The figure shows three views and two pictorial views of one solid part (mm, origin at its lowest corner). Answer the questions. A direction names the side the tool comes from. Coordinates: 2 decimals unless noted, no trailing zeros. Loops run counter-clockwise (first coordinate to the right, second up) from the corner with the lowest first, then second, coordinate; pieces in that order, holes last. Notation, with made-up numbers: M 16.5,74 L 31.5,74 A32 ccw 31.5,102 Z; hole C 49,-26.5 d10. An arc over 180 degrees is marked long. Answer as a JSON object with one key per item and string values. Group by question number.
1. A cutting plane is placed at B-B on y = 2. Give the vertices of the cut face in (x, z), and give its area (3 significant figures).
2. For the marked faces 1 and 2, determine the directions among +Z, -Z, +X, -X, +Y, -Y from which every point of the face is accessible in a straight line to the end or side of a thin tool.
3. A cutting plane is placed at A-A on y = 8.25. Give the vertices of the cut face in (x, z).
4. Straight lines are drawn through the part: L1, parallel to Y at x = 2.85, z = 1.65; L2, parallel to X at y = 5, z = 1.55; L3, parallel to X at y = 3, z = 1. For each, find the intervals that lie inside material, in ascending order.
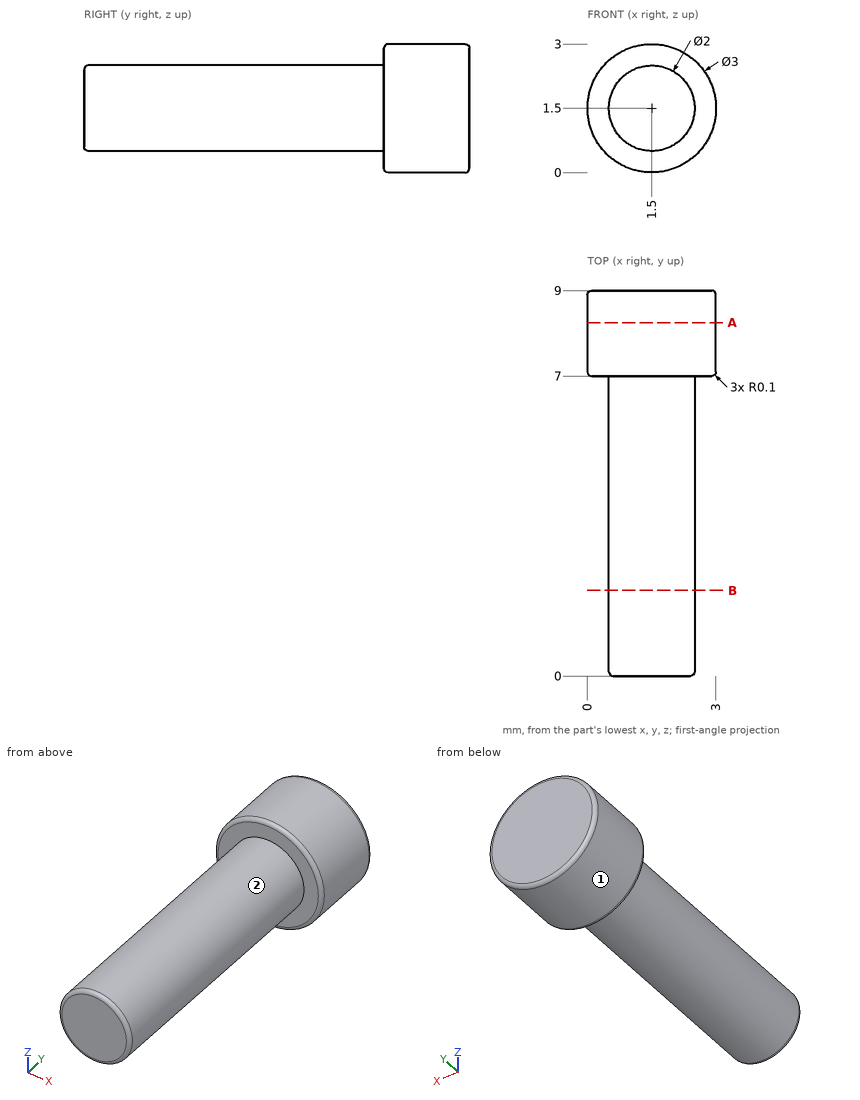
From the geometry:
{
 "1": {"outline": "C 1.5,1.5 d2", "area": "3.14 mm²"},
 "2": {"face 1": "+Y, -Y", "face 2": "-Y"},
 "3": {"outline": "C 1.5,1.5 d3"},
 "4": {"L1": "y = 7 to 9", "L2": "x = 0.5 to 2.5", "L3": "x = 0.63 to 2.37"}
}
